```python
from build123d import *

# Parameters (mm, degrees)
SKETCH1_W           = 34.5
SKETCH1_H           = 20
BOSS_EXTRUDE1_DEPTH = 9
CUT_EXTRUDE1_DEPTH  = 6
SKETCH5_W           = 3
SKETCH5_H           = 4
CUT_EXTRUDE2_DEPTH  = 35
SKETCH7_W           = 2.7
SKETCH7_H           = 4.2
BOSS_EXTRUDE3_DEPTH = 3
SKETCH14_R          = 0.75
CUT_EXTRUDE9_DEPTH  = 2
SKETCH8_R           = 1.25
SKETCH8_W           = 9
SKETCH8_H           = 1.1
CUT_EXTRUDE3_DEPTH  = 5
CHAMFER1_SIZE       = 1.4
CHAMFER1_SIZE_2     = 7.202375622
SKETCH6_W           = 31.5
SKETCH6_H           = 5
CUT_EXTRUDE6_DEPTH  = 2
SKETCH11_W          = 2.6
SKETCH11_H          = 2.8
CUT_EXTRUDE7_DEPTH  = 2
SKETCH12_W          = 3
SKETCH12_H          = 3
CUT_EXTRUDE8_DEPTH  = 7
SKETCH16_W          = 7.95
SKETCH16_H          = 3.1
CUT_EXTRUDE10_DEPTH = 2
SKETCH17_W          = 7.95
SKETCH17_H          = 7
CUT_EXTRUDE11_DEPTH = 1.5
SKETCH18_W          = 1.5
SKETCH18_H          = 5
CUT_EXTRUDE12_DEPTH = 2
SKETCH20_W          = 22.05
SKETCH20_H          = 3.75
CUT_EXTRUDE13_DEPTH = 7
SKETCH21_W          = 7.2
SKETCH21_H          = 2.75
CUT_EXTRUDE14_DEPTH = 5


with BuildPart() as part:
    # Sketch1 → Boss-Extrude1 (new body)
    with BuildSketch(Plane.XY):
        Rectangle(SKETCH1_W, SKETCH1_H)
    extrude(amount=BOSS_EXTRUDE1_DEPTH)

    # Sketch3 → Cut-Extrude1 (cut)
    with BuildSketch(Plane.XY.offset(9)):
        Polygon((15.7, -6.9), (15.7, 3.1), (-9.3, 3.1), (-9.3, 6.9), (-15.7, 6.9), (-15.7, -6.9), align=None)
    extrude(amount=-CUT_EXTRUDE1_DEPTH, mode=Mode.SUBTRACT)

    # Sketch5 → Cut-Extrude2 (cut)
    with BuildSketch(Plane(origin=(17.25, 0, 0), x_dir=(0, 0, -1), z_dir=(1, 0, 0))):
        with Locations((-1.5, 0)):
            Rectangle(SKETCH5_W, SKETCH5_H)
    extrude(amount=-CUT_EXTRUDE2_DEPTH, mode=Mode.SUBTRACT)

    # Sketch7 → Boss-Extrude3 (add)
    with BuildSketch(Plane.XY.offset(3)):
        with Locations((-14.35, 4.8)):
            Rectangle(SKETCH7_W, SKETCH7_H)
    extrude(amount=BOSS_EXTRUDE3_DEPTH)

    # Sketch14 → Cut-Extrude9 (cut)
    with BuildSketch(Plane.XY.offset(3)):
        with Locations((-11, 5.3)):
            Circle(SKETCH14_R)
    extrude(amount=-CUT_EXTRUDE9_DEPTH, mode=Mode.SUBTRACT)

    # Sketch8 → Cut-Extrude3 (cut)
    with BuildSketch(Plane.XY.offset(9)):
        with Locations((14.149147106, 4.8)):
            Circle(SKETCH8_R)
        with Locations((-10.85, -7.45)):
            Rectangle(SKETCH8_W, SKETCH8_H)
        with Locations((10.85, -7.45)):
            Rectangle(SKETCH8_W, SKETCH8_H)
    extrude(amount=-CUT_EXTRUDE3_DEPTH, mode=Mode.SUBTRACT)

    # Chamfer1
    # the kernel refuses this chamfer: 7.202375622, 1.4 mm, written as the material it takes off along each edge
    with BuildSketch(Plane(origin=(-15.7, 6.9, 9), x_dir=(-0.9816291836389949, 0, 0.190798704996235), z_dir=(0, -1, 0))) as chamfer1_piece_1_section:
        Polygon((CHAMFER1_SIZE * 0.981629183639, CHAMFER1_SIZE * 0.190798704996), (-CHAMFER1_SIZE_2 * 0.190798705006, CHAMFER1_SIZE_2 * 0.981629183688), (0, 0), align=None)
    chamfer1_piece_1 = extrude(amount=13.8, mode=Mode.PRIVATE)
    chamfer1_piece_1 = split(chamfer1_piece_1, bisect_by=Plane(origin=(-16.266997619, 4.8, 6), z_dir=(0, 0, 1)), keep=Keep.TOP, mode=Mode.PRIVATE)
    add(chamfer1_piece_1, mode=Mode.SUBTRACT)
    with BuildSketch(Plane(origin=(-15.7, 25.613448453, 9), x_dir=(-0.9816291836389951, 0, 0.19079870499623477), z_dir=(0, -1, 0))) as chamfer1_piece_2_section:
        Polygon((CHAMFER1_SIZE * 0.981629183639, CHAMFER1_SIZE * 0.190798704996), (-CHAMFER1_SIZE_2 * 0.190798705006, CHAMFER1_SIZE_2 * 0.981629183688), (0, 0), align=None)
    chamfer1_piece_2 = extrude(amount=32.513448453, mode=Mode.PRIVATE)
    chamfer1_piece_2 = split(chamfer1_piece_2, bisect_by=Plane(origin=(-15.989617837, 2.35, 3), z_dir=(0, 0, 1)), keep=Keep.TOP, mode=Mode.PRIVATE)
    chamfer1_piece_2 = split(chamfer1_piece_2, bisect_by=Plane(origin=(-15.989617837, 2.7, 4.777533587), z_dir=(0, -1, 0)), keep=Keep.TOP, mode=Mode.PRIVATE)
    add(chamfer1_piece_2, mode=Mode.SUBTRACT)

    # Sketch6 → Cut-Extrude6 (cut)
    with BuildSketch(Plane(origin=(0, 0, 0), x_dir=(-1, 0, 0), z_dir=(0, 0, -1))):
        with Locations((0, 6)):
            Rectangle(SKETCH6_W, SKETCH6_H)
        with Locations((0, -6)):
            Rectangle(SKETCH6_W, SKETCH6_H)
    extrude(amount=-CUT_EXTRUDE6_DEPTH, mode=Mode.SUBTRACT)

    # Sketch11 → Cut-Extrude7 (cut)
    with BuildSketch(Plane(origin=(17.25, 0, 0), x_dir=(0, 0, -1), z_dir=(1, 0, 0))):
        with Locations((-4.3, -0.9)):
            Rectangle(SKETCH11_W, SKETCH11_H)
    extrude(amount=-CUT_EXTRUDE7_DEPTH, mode=Mode.SUBTRACT)

    # Sketch12 → Cut-Extrude8 (cut)
    with BuildSketch(Plane(origin=(0, 0, 2), x_dir=(-1, 0, 0), z_dir=(0, 0, -1))):
        with Locations((4.25, 7)):
            Rectangle(SKETCH12_W, SKETCH12_H)
    extrude(amount=-CUT_EXTRUDE8_DEPTH, mode=Mode.SUBTRACT)

    # Sketch16 → Cut-Extrude10 (cut)
    with BuildSketch(Plane.XY.offset(9)):
        with Locations((-13.275, 8.45)):
            Rectangle(SKETCH16_W, SKETCH16_H)
    extrude(amount=-CUT_EXTRUDE10_DEPTH, mode=Mode.SUBTRACT)

    # Sketch17 → Cut-Extrude11 (cut)
    with BuildSketch(Plane(origin=(0, 10, 0), x_dir=(1, 0, 0), z_dir=(0, 1, 0))):
        with Locations((-13.275, -3.5)):
            Rectangle(SKETCH17_W, SKETCH17_H)
    extrude(amount=-CUT_EXTRUDE11_DEPTH, mode=Mode.SUBTRACT)

    # Sketch18 → Cut-Extrude12 (cut)
    with BuildSketch(Plane.XY):
        with Locations((-16.5, 6)):
            Rectangle(SKETCH18_W, SKETCH18_H)
    extrude(amount=CUT_EXTRUDE12_DEPTH, mode=Mode.SUBTRACT)

    # Sketch20 → Cut-Extrude13 (cut)
    with BuildSketch(Plane(origin=(0, 0, 0), x_dir=(-1, 0, 0), z_dir=(0, 0, -1))):
        with Locations((-1.725, 3.875)):
            Rectangle(SKETCH20_W, SKETCH20_H)
    extrude(amount=-CUT_EXTRUDE13_DEPTH, mode=Mode.SUBTRACT)

    # Sketch21 → Cut-Extrude14 (cut)
    with BuildSketch(Plane(origin=(0, 0, 2), x_dir=(-1, 0, 0), z_dir=(0, 0, -1))):
        with Locations((4.25, 7.125)):
            Rectangle(SKETCH21_W, SKETCH21_H)
    extrude(amount=-CUT_EXTRUDE14_DEPTH, mode=Mode.SUBTRACT)


solid = part.part
```
Build history of the part. All positions in model axes, mm. A direction names the side the tool comes from. Round coordinates to 2 decimals unless told otherwise and drop trailing zeros. Write each loop counter-clockwise with the first axis right and the second up, starting at its lowest first coordinate (ties: lowest second). Pieces come first, ordered by that corner, then holes.
1) Pin check, flat tips, straight feed: pin 1 (1.5 mm diameter, centred on x = -12.5, z = 5.5, fed in from +Y); pin 2 (12 mm diameter, centred on x = -9, y = -6.5, fed in from +Z); pin 3 (2 mm diameter, centred on x = 14.15, y = 4.8, fed in from +Z). Stop position of each tip, or through.
2) Band-saw the part on D-D, the plane x = -5. List the corners of the cut face in (y, z).
3) Band-saw the part on C-C, the plane x = 9. List the corners of the cut face in (y, z), and give its area (4 significant figures).
4) Band-saw the part on B-B, the plane y = 1. List the corners of the cut face in (x, z).
5) Drill centre lines: probe 1 along Y at (x, z) = (-11, 2.35); probe 2 along Y at (x, z) = (0.5, 1); probe 3 along Y at (x, z) = (-14, 5). Where is each one in solid material? Low to high.
6) Mould opens along Y. For faces 1 (the flat face through (16, 1, 3)), 2 (the flat face through (0, -9, 0)), 3 (the flat face through (4, 10, 4)) say: +Y half, -Y half, draft (parallel to the pull), parting line (faces both ways), or undercut.
7) 3-axis set-ups, long thin cutter, end or side, ignore diameter. For faces 4 (the flat face through (12.75, 4, 3)), 5 (the flat face through (9, 7, 2)), 6 (the flat face through (17.25, 0, 6)), 7 (the flat face through (-13, 5, 4)), 8 (the flat face through (-17.25, -1, 4)): which of +Z, -Z, +X, -X, +Y, -Y reach the whole face in a straight line?
8) Band-saw the part on A-A, the plane z = 2.5. List the corners of the cut face in (x, y).
Ans:
1. pin 1: stops at y = 8.5
1. pin 2: stops at z = 9
1. pin 3: stops at z = 4
2. outline: (-10, 0) - (-8.5, 0) - (-8.5, 2) - (-3.5, 2) - (-3.5, 0) - (-2, 0) - (-2, 3) - (-6.9, 3) - (-6.9, 9) - (-10, 9) - close; (3.1, 7) - (5.5, 7) - (5.5, 9) - (3.1, 9) - close; (8.5, 0) - (10, 0) - (10, 9) - (8.5, 9) - close
3. outline: (-10, 0) - (-8.5, 0) - (-8.5, 2) - (-3.5, 2) - (-3.5, 0) - (-2, 0) - (-2, 3) - (-6.9, 3) - (-6.9, 4) - (-8, 4) - (-8, 9) - (-10, 9) - close; (3.1, 7) - (5.75, 7) - (5.75, 2) - (8.5, 2) - (8.5, 0) - (10, 0) - (10, 9) - (3.1, 9) - close
3. area: 65.15 mm2
4. outline: (-17.25, 3) - (-15.93, 3) - (-17.1, 9) - (-17.25, 9) - close; (15.7, 3) - (17.25, 3) - (17.25, 9) - (15.7, 9) - close
5. probe 1: y = -10 to -2, 2 to 4.55, 6.05 to 8.5
5. probe 2: y = -10 to -8.5, -3.5 to -2, 8.5 to 10
5. probe 3: y = -10 to -8, 2.7 to 8.5
6. face 1: undercut
6. face 2: draft
6. face 3: +Y half
7. face 4: -Z
7. face 5: -Z, -X
7. face 6: +Z, -Z, +X, +Y, -Y
7. face 7: +Z
7. face 8: +Z, -Z, -X, +Y, -Y
8. outline: (-17.25, -10) - (17.25, -10) - (17.25, -2) - (-17.25, -2) - close; (-17.25, 2) - (-9.3, 2) - (-9.3, 5.75) - (-7.85, 5.75) - (-7.85, 8.5) - (-0.65, 8.5) - (-0.65, 5.75) - (12.75, 5.75) - (12.75, 2) - (17.25, 2) - (17.25, 10) - (-9.3, 10) - (-9.3, 8.5) - (-17.25, 8.5) - close; hole circle Ø1.5 at (-11, 5.3)
